Verification items for the finished model (mm, model axes). Give positions to 0.01 mm unless a question says otherwise; leave off trailing zeros. Write each loop counter-clockwise with the first axis right and the second up, starting at its lowest first coordinate (ties: lowest second). Pieces come first, ordered by that corner, then holes. Notation, with made-up numbers: M 68,60.5 L 122,60.5 A21 cw 122,67.5 Z; hole C 4,16.25 d7. An arc over 180 degrees is marked long. Answer as a JSON object with one key per item and string values.
```python
from build123d import *

# Parameters (mm, degrees)
SKETCH1_W              = 19.05
SKETCH1_H              = 19.05
SKETCH1_W_2            = 12.7
SKETCH1_H_2            = 12.7
BOSS_EXTRUDE1_DEPTH    = 431.8
CUT_EXTRUDE1_DEPTH     = 20.05
F_10_CLEARANCE_HOLE1_D = 5.1054


with BuildPart() as part:
    # Sketch1 → Boss-Extrude1 (new body)
    with BuildSketch(Plane(origin=(0, 0, 0), x_dir=(0, 0, -1), z_dir=(1, 0, 0))):
        with Locations((9.525, 9.525)):
            Rectangle(SKETCH1_W, SKETCH1_H)
        with Locations((9.525, 9.525)):
            Rectangle(SKETCH1_W_2, SKETCH1_H_2, mode=Mode.SUBTRACT)
    extrude(amount=BOSS_EXTRUDE1_DEPTH)

    # Sketch2 → Cut-Extrude1 (cut, through all)
    with BuildSketch(Plane.XY):
        Polygon((398.348522628, 19.05), (409.347045256, 0), (431.8, 0), (431.8, 19.05), align=None)
        Polygon((0, 19.05), (0, 0), (10.998522628, 19.05), align=None)
    extrude(amount=-CUT_EXTRUDE1_DEPTH, mode=Mode.SUBTRACT)

    # #10 Clearance Hole1 (through all)
    with Locations(Plane(origin=(368.072045256, 9.525, 0), x_dir=(1, 0, 0), z_dir=(0, 0, 1))):
        with Locations((0, 0), (-326.797045256, 0)):
            Hole(F_10_CLEARANCE_HOLE1_D / 2)


solid = part.part
```
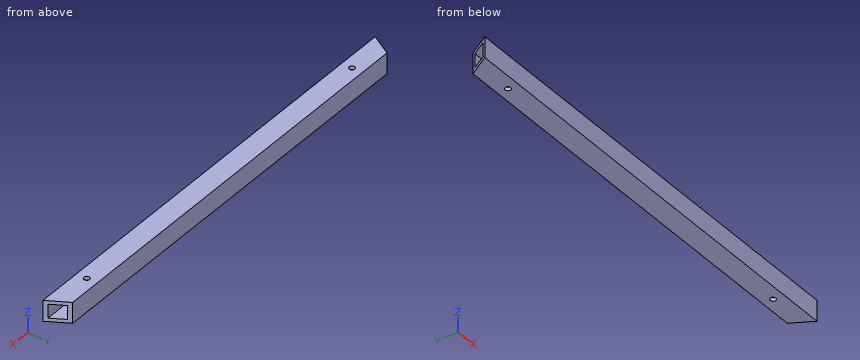
1) Go/stop test with a flat-tipped pin: pin 1 (6 mm diameter, centred on x = 41.275, y = 9.525, fed in from +Z). Record where the tip stops, or that it passes through.
Completed:
{"pin 1": "stops at z = 0"}
2) Section check B-B on z = -10.5. Record the boundary of the cut face in (x, y) (3 decimals), and give its area (3 significant figures).
Completed:
{"outline": "M 0,0 L 409.347,0 L 407.514,3.175 L 1.833,3.175 Z; M 9.165,15.875 L 400.182,15.875 L 398.349,19.05 L 10.999,19.05 Z", "area": "2,530 mm2"}
3) Section check A-A on x = 116. Record the boundary of the cut face in (y, z) (3 decimals).
Completed:
{"outline": "M 0,-19.05 L 19.05,-19.05 L 19.05,0 L 0,0 Z; hole M 3.175,-15.875 L 15.875,-15.875 L 15.875,-3.175 L 3.175,-3.175 Z"}
4) Thickness scan on L1, parallel to Y at x = 356.5, z = -15 (3 decimals); L2, parallel to Z at x = 273, y = 5.75 (3 decimals); L3, parallel to X at y = 18.25, z = -14.25. Record the ranges inside material, lowest first.
Completed:
{"L1": "y = 0 to 3.175, 15.875 to 19.05", "L2": "z = -19.05 to -15.875, -3.175 to 0", "L3": "x = 10.54 to 398.81"}
